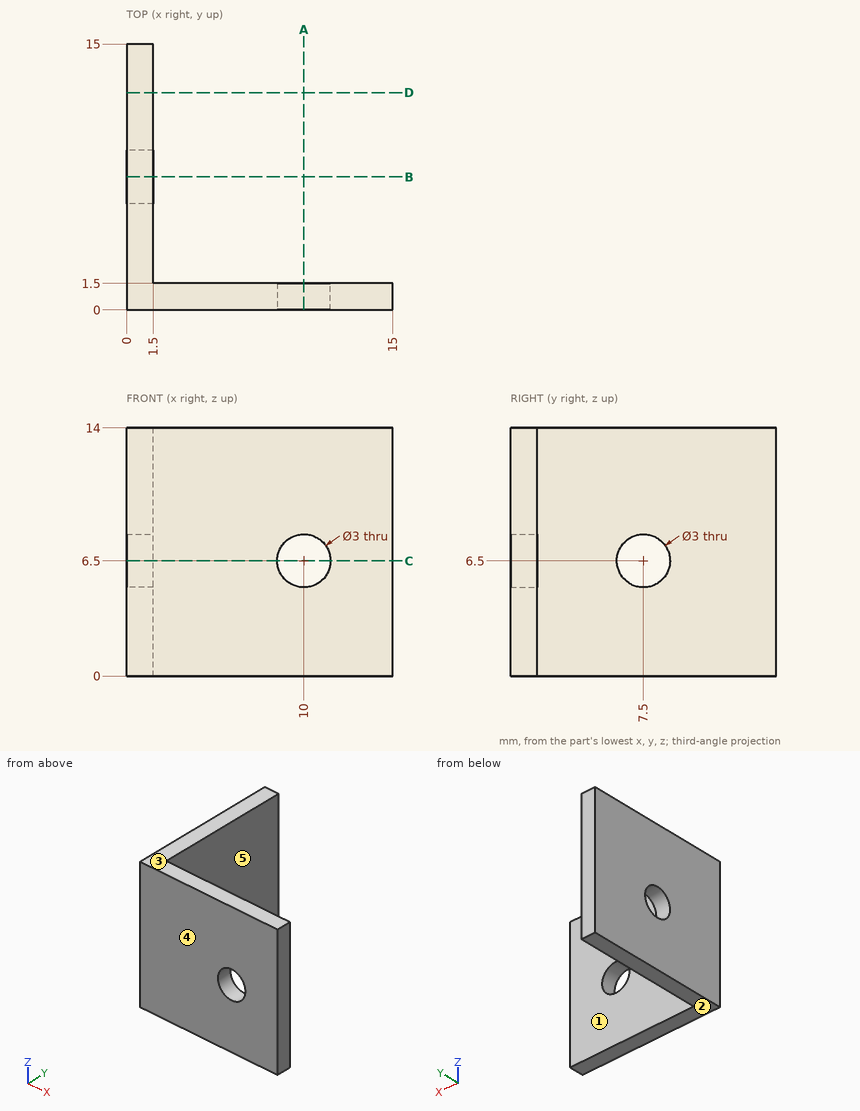
Design review of the part shown in the three views and the two pictorial views. Dimensions are in mm from the part's minimum x, y and z. A direction names the side the tool comes from. Coordinates: 2 decimals unless noted, no trailing zeros. Write each loop counter-clockwise with the first axis right and the second up, starting at its lowest first coordinate (ties: lowest second). Pieces come first, ordered by that corner, then holes. Notation, with made-up numbers: (67, -27.75) -> (98, -27.75) arc R19 ccw to (98, 5.25) -> close; hole circle Ø10 at (89, -35). An arc over 180 degrees is marked (long way). Answer in a Markdown table with one row per item.
1. We need section A-A, the plane x = 10. State the section outline as (y, z) points, and give its area (3 significant figures).
Answers below:
| item | result |
|---|---|
| outline | (0, 0) -> (1.5, 0) -> (1.5, 5) -> (0, 5) -> close; (0, 8) -> (1.5, 8) -> (1.5, 14) -> (0, 14) -> close |
| area | 16.5 mm^2 |
2. We need section C-C, the plane z = 6.5. State the section outline as (x, y) points, and give its area (4 significant figures).
Answers below:
| item | result |
|---|---|
| outline | (0, 0) -> (8.5, 0) -> (8.5, 1.5) -> (1.5, 1.5) -> (1.5, 6) -> (0, 6) -> close; (0, 9) -> (1.5, 9) -> (1.5, 15) -> (0, 15) -> close; (11.5, 0) -> (15, 0) -> (15, 1.5) -> (11.5, 1.5) -> close |
| area | 33.75 mm^2 |
3. Wall thickness on probe 1 along Y at (x, z) = (0.4, 6.5); probe 2 along Z at (x, y) = (10, 0.65); probe 3 along X at (y, z) = (3, 2.5): over which ranges is each line inside the solid? List them lowest first. Write a range as [from, to].
Answers below:
| item | result |
|---|---|
| probe 1 | y = [0, 6], [9, 15] |
| probe 2 | z = [0, 5], [8, 14] |
| probe 3 | x = [0, 1.5] |
4. Draft analysis for pull direction Z (two halves, no side actions). For the marked faces 1, 2 and 3, state which applies: +Z half, -Z half, draft (parallel to the pull), parting line (faces both ways), or undercut.
Answers below:
| item | result |
|---|---|
| face 1 | draft |
| face 2 | -Z half |
| face 3 | +Z half |
5. Clearance check with flat-ended pins moving along their axes: pin 1 Ø5 at (x, y) = (5, 7.5) entering from -Z; pin 2 Ø6 at (x, z) = (13, 10) entering from +Y; pin 3 Ø4 at (y, z) = (7.5, 4.5) entering from +X. State where each tip first meets the part, or that it passes through.
Answers below:
| item | result |
|---|---|
| pin 1 | passes through |
| pin 2 | stops at y = 1.5 |
| pin 3 | stops at x = 1.5 |
6. We need section D-D, the plane y = 12.25. State the section outline as (x, z) points.
Answers below:
| item | result |
|---|---|
| outline | (0, 0) -> (1.5, 0) -> (1.5, 14) -> (0, 14) -> close |
7. For the marked faces 4 and 5, list the 3-axis set-ups (+Z, -Z, +X, -X, +Y, -Y) from which the entire face can be reached by the end or side of a thin tool; tool diameter is ignored.
Answers below:
| item | result |
|---|---|
| face 4 | +Z, -Z, +X, -X, -Y |
| face 5 | +Z, -Z, +X, +Y |
